Can you work these out from the drawing? Everything is in mm from the part's minimum corner. Coordinates: 2 decimals unless noted, no trailing zeros. Loops run counter-clockwise (first coordinate to the right, second up) from the corner with the lowest first, then second, coordinate; pieces in that order, holes last. Notation, with made-up numbers: (61, 43) -> (86, 43) arc R20 cw to (86, 70) -> close; hole circle Ø7 at (48.5, 89.5). An arc over 180 degrees is marked (long way). One line per question, with ' | ' between items.
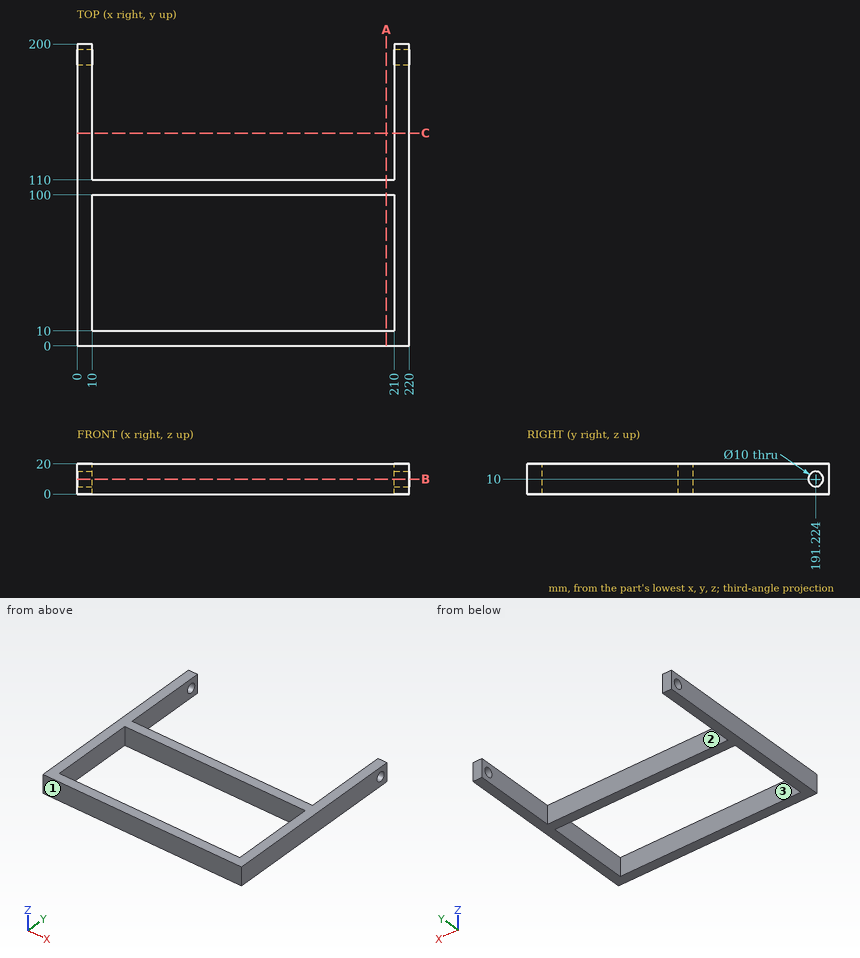
Q1. We'd pull the mould along X, two halves only. Please class the marked faces 1, 2 and 3: released by +X, released by -X, zero draft, split by the parting line, or undercut.
Values follow:
face 1: zero draft | face 2: undercut | face 3: undercut
Q2. Imagine slicing it at C-C on y = 141. Write out the boundary of the cut face in (x, z), plus the area to 3 significant figures.
Values follow:
outline: (0, 0) -> (10, 0) -> (10, 20) -> (0, 20) -> close; (210, 0) -> (220, 0) -> (220, 20) -> (210, 20) -> close | area: 400 mm2
Q3. Imagine slicing it at B-B on z = 10. Write out the boundary of the cut face in (x, y) (1 decimal), plus the area to 3 significant figures.
Values follow:
outline: (0, 0) -> (220, 0) -> (220, 186.2) -> (210, 186.2) -> (210, 110) -> (10, 110) -> (10, 186.2) -> (0, 186.2) -> close; (0, 196.2) -> (10, 196.2) -> (10, 200) -> (0, 200) -> close; (210, 196.2) -> (220, 196.2) -> (220, 200) -> (210, 200) -> close; hole (10, 10) -> (210, 10) -> (210, 100) -> (10, 100) -> close | area: 7,800 mm2
Q4. For pin 1 (9 mm diameter, centred on y = 191.22, z = 10, fed in from -X); pin 2 (10 mm diameter, centred on x = 85.5, z = 15, fed in from +Y), each with a flat end and sliding along its axis, tell me the tip position at first contact or that it passes through.
Values follow:
pin 1: passes through | pin 2: stops at y = 110
Q5. Imagine slicing it at A-A on x = 205. Write out the boundary of the cut face in (y, z), plus the area to 3 significant figures.
Values follow:
outline: (0, 0) -> (10, 0) -> (10, 20) -> (0, 20) -> close; (100, 0) -> (110, 0) -> (110, 20) -> (100, 20) -> close | area: 400 mm2
Q6. Please list where these lines run through material, in increasing order: L1, parallel to X at y = 119, z = 13.5; L2, parallel to Y at x = 185.5, z = 11.75. Write a range as [from, to].
Values follow:
L1: x = [0, 10], [210, 220] | L2: y = [0, 10], [100, 110]
